Check sheet for the drawn part. Datum: minimum x, y, z corner. Units: mm. A direction names the side the tool comes from. Round coordinates to 2 decimals unless told otherwise and drop trailing zeros. Write each loop counter-clockwise with the first axis right and the second up, starting at its lowest first coordinate (ties: lowest second). Pieces come first, ordered by that corner, then holes.
Item 1: Tool access check on the marked faces 4 and 5. Record the directions out of +Z, -Z, +X, -X, +Y, -Y that give a thin tool (end or side, any length) a straight path to the whole face; none if there is none.
Item 2: Cross-section at D-D on z = 40. Enter the section's corners in (x, y).
Item 3: Cross-section at A-A on z = 23.5. Enter the section's corners in (x, y), plus the area to 3 significant figures.
Item 4: Material ranges on line 1 (X direction, y = 6, z = 19); line 2 (Z direction, x = 37.5, y = 19.15); line 3 (X direction, y = 18.85, z = 23.5), recorded low to high.
Item 5: Cross-section at C-C on y = 16. Enter the section's corners in (x, z), plus the area to 3 significant figures.
Item 6: Release check for a two-part mould opening along X. For the marked faces 1, 2 and 3 record: +X half, -X half, draft (parallel to the pull), parting line (faces both ways), or undercut.
Item 7: Cross-section at B-B on x = 37.5. Enter the section's corners in (y, z).
Item 8: Go/stop test with a flat-tipped pin: pin 1 Ø8 at (x, z) = (25, 13) entering from -Y. Record where the tip stops, or that it passes through.
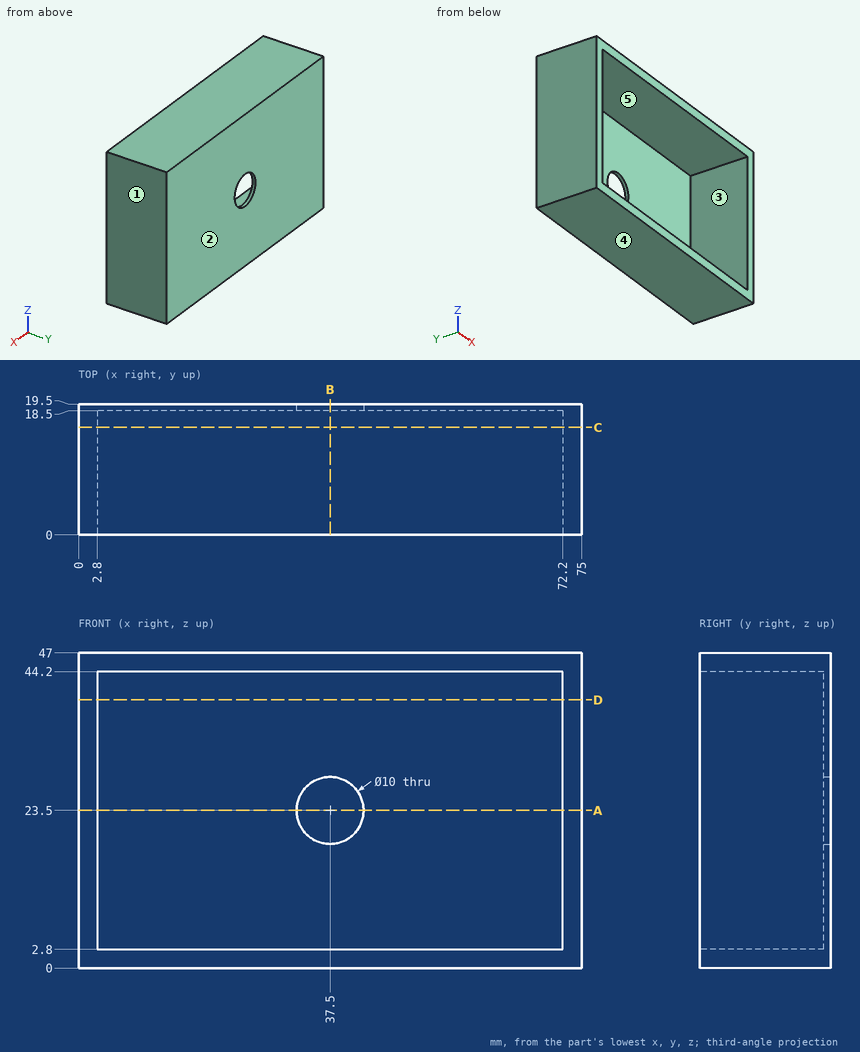
Response values:
1. face 4: -Z, +X, -X, +Y, -Y
1. face 5: -Y
2. outline: (0, 0) - (2.8, 0) - (2.8, 18.5) - (72.2, 18.5) - (72.2, 0) - (75, 0) - (75, 19.5) - (0, 19.5) - close
3. outline: (0, 0) - (2.8, 0) - (2.8, 18.5) - (32.5, 18.5) - (32.5, 19.5) - (0, 19.5) - close; (42.5, 18.5) - (72.2, 18.5) - (72.2, 0) - (75, 0) - (75, 19.5) - (42.5, 19.5) - close
3. area: 169 mm2
4. line 1: x = 0 to 2.8, 72.2 to 75
4. line 2: z = 0 to 18.5, 28.5 to 47
4. line 3: x = 0 to 32.5, 42.5 to 75
5. outline: (0, 0) - (75, 0) - (75, 47) - (0, 47) - close; hole (2.8, 2.8) - (72.2, 2.8) - (72.2, 44.2) - (2.8, 44.2) - close
5. area: 652 mm2
6. face 1: +X half
6. face 2: draft
6. face 3: undercut
7. outline: (0, 0) - (19.5, 0) - (19.5, 18.5) - (18.5, 18.5) - (18.5, 2.8) - (0, 2.8) - close; (0, 44.2) - (18.5, 44.2) - (18.5, 28.5) - (19.5, 28.5) - (19.5, 47) - (0, 47) - close
8. pin 1: stops at y = 18.5
